Could you check a few things on this model? Use its own coordinates, in mm. Face numbers are marked on the shaded views. A direction names the side the tool comes from. Round coordinates to 2 decimals unless told otherwise and drop trailing zeros. Loops run counter-clockwise (first coordinate to the right, second up) from the corner with the lowest first, then second, coordinate; pieces in that order, holes last. Notation, with made-up numbers: (63.25, 13) -> (122.25, 13) arc R17 cw to (122.25, 46) -> close; hole circle Ø4 at (50, 1). An arc over 180 degrees is marked (long way). Write each question's results on one line, items separated by ' | '. Start each with the question number.
1) Imagine slicing it at B-B, the plane z = 7.25. List the corners of the cut face in (x, y) for me, plus the area to 3 significant figures.
2) Imagine slicing it at D-D, the plane x = 6.5. List the corners of the cut face in (y, z) for me.
3) For P1, Ø0.6, axis at x = -5, y = 7, coming from the +Z side; P2, Ø8, axis at y = 1.5, z = 8.5, coming from the -X side; P3, Ø5, axis at x = 0, z = 10.52, coming from the +Y side; P4, Ø4, axis at x = -20.5, z = 8.5, coming from the +Y side, each with a flat end and sliding along its axis, tell me the tip position at first contact or that it passes through.
4) Imagine slicing it at C-C, the plane y = -4.75. List the corners of the cut face in (x, z) for me.
5) If I drill on probe 1 along Z at (x, y) = (0, -3); probe 2 along X at (y, z) = (-0.25, 7); probe 3 along Y at (x, z) = (5, 12.5), over which ranges is the centre line in solid material (lowest first)?
6) Imagine slicing it at A-A, the plane x = 0. List the corners of the cut face in (y, z) for me.
7) We'd pull the mould along Z, two halves only. Please class the marked faces 3, 4 and 5: pulls with the +Z half, pulls with the -Z half, needs draft (parallel to the pull), parting line crosses it, or undercut.
8) Which directions (+Z, -Z, +X, -X, +Y, -Y) give clear straight access to the entire face, cutting with the end or side of a thin tool? Please do the marked faces 1 and 2.
from build123d import *

# Parameters (mm, degrees)
F0_R        = 4.1158301742
F1_DEPTH    = 6.35
F0_W        = 54.6039827168
F0_H        = 10.6174414977
F2_DEPTH    = 12.7
F3_T1_DEPTH = 80.7322818745
F3_T3_DEPTH = 29.5163540068
F3_T5_DEPTH = 29.5163538598


# Not quite as in the source:
# - a fillet or chamfer that OpenCascade refuses, or shapes differently, is made with other operations: its cross-section is extruded or revolved along the edge and cut away or added


with BuildPart() as f1:
    # F0 (on Front) → F1 (new body, symmetric)
    with BuildSketch(Plane.XZ):
        Polygon((-5.6879152544, 15.7365649939), (-27.3019913584, 5.3087207489), (27.3019913584, 5.3087207489), (5.68791572, 15.7365649939), (0, 15.7365649939), align=None)
        with Locations((0, 10.5226428714)):
            Circle(F0_R, mode=Mode.SUBTRACT)
    extrude(amount=F1_DEPTH, both=True)

    # F0 (on Front) → F2 (join, symmetric)
    with BuildSketch(Plane.XZ):
        Rectangle(F0_W, F0_H)
    extrude(amount=F2_DEPTH, both=True)

    # F3: chamfer of 5.08 on 4 edges, made by hand

    # F3_s2 → F3_t1 (cut)
    with BuildSketch(Plane.YZ.offset(-40.3661409373)):
        Polygon((-7.62, 5.3087207489), (-12.7, 0.2287207489), (-12.7, 5.3087207489), align=None)
        Polygon((7.62, 5.3087207489), (12.7, 0.2287207489), (12.7, 5.3087207489), align=None)
    extrude(amount=F3_T1_DEPTH, mode=Mode.SUBTRACT)

    # F3_s4 → F3_t3 (cut)
    with BuildSketch(Plane.XZ.offset(-14.7581770034)):
        Polygon((-27.3019913584, 2.1192789571), (-24.4293942586, 6.6946229263), (-27.3019913584, 5.3087207489), align=None)
    extrude(amount=F3_T3_DEPTH, mode=Mode.SUBTRACT)

    # F3_s6 → F3_t5 (cut)
    with BuildSketch(Plane.XZ.offset(-14.7581769299)):
        Polygon((27.3019913584, 2.119278987), (24.4293942972, 6.6946229375), (27.3019913584, 5.3087207489), align=None)
    extrude(amount=F3_T5_DEPTH, mode=Mode.SUBTRACT)


solid = f1.part
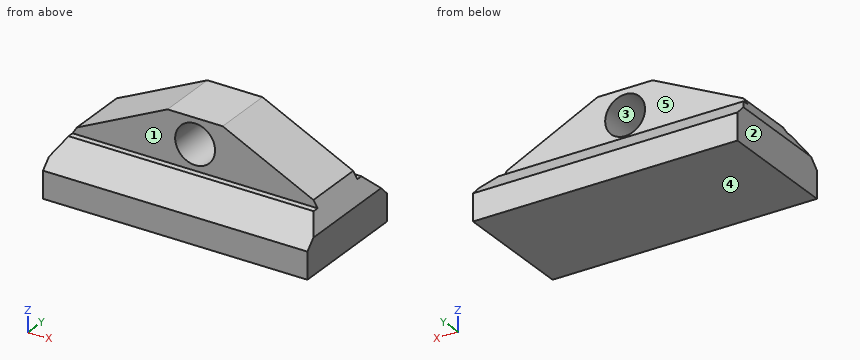
Checked values:
1) outline: (-23.28, -6.35) -> (-2.5, -6.35) -> (-2.5, 6.35) -> (-23.28, 6.35) -> close; (2.5, -6.35) -> (23.28, -6.35) -> (23.28, 6.35) -> (2.5, 6.35) -> close | area: 528 mm^2
2) outline: (-12.7, -5.31) -> (12.7, -5.31) -> (12.7, 0.23) -> (7.62, 5.31) -> (6.35, 5.31) -> (6.35, 15.34) -> (-6.35, 15.34) -> (-6.35, 5.31) -> (-7.62, 5.31) -> (-12.7, 0.23) -> close
3) P1: z = 5.31 | P2: x = -25.81 | P3: through | P4: y = 6.35
4) outline: (-27.3, -5.31) -> (27.3, -5.31) -> (27.3, 2.12) -> (24.43, 6.69) -> (5.69, 15.74) -> (-5.69, 15.74) -> (-24.43, 6.69) -> (-27.3, 2.12) -> close; hole circle Ø8.23 at (0, 10.52)
5) probe 1: -5.31 to 6.41, 14.64 to 15.74 | probe 2: -23.8 to -2.13, 2.13 to 23.8 | probe 3: -6.35 to 6.35
6) outline: (-12.7, -5.31) -> (12.7, -5.31) -> (12.7, 0.23) -> (7.62, 5.31) -> (6.35, 5.31) -> (6.35, 6.41) -> (-6.35, 6.41) -> (-6.35, 5.31) -> (-7.62, 5.31) -> (-12.7, 0.23) -> close; (-6.35, 14.64) -> (6.35, 14.64) -> (6.35, 15.74) -> (-6.35, 15.74) -> close
7) face 3: undercut | face 4: pulls with the -Z half | face 5: needs draft
8) face 1: +Z, +X, -X, -Y | face 2: +Z, -Z, -X, +Y, -Y
